from build123d import *

# Parameters (mm, degrees)
BOSS_EXTRUDE1_DEPTH = 2.5


with BuildPart() as part:
    # Sketch1 → Boss-Extrude1 (new, symmetric)
    with BuildSketch(Plane.XY):
        with BuildLine():
            Line((-25, 0), (-25, -40))
            Line((-25, -40), (25, -40))
            Line((25, -40), (25, 0))
            Line((25, 0), (18, 0))
            ThreePointArc((18, 0), (0, -18), (-18, 0))
            Line((-18, 0), (-25, 0))
        make_face()
    extrude(amount=BOSS_EXTRUDE1_DEPTH, both=True)


solid = part.part
Here's how the part is built. I have some questions about the finished solid (model axes, mm). Round coordinates to 2 decimals unless told otherwise and drop trailing zeros. Order: outer loops, then holes, each group sorted by start corner. A loop starts at its lowest first (then second) coordinate and runs counter-clockwise, first axis right, second up. Notation, with made-up numbers: (69, 19.25) -> (94, 19.25) arc R21 cw to (94, 28.25) -> close; hole circle Ø3 at (12, 46.5). An arc over 180 degrees is marked (long way). Return JSON: item names as keys, results as strings.
Q1. If we section it at B-B on z = -0.7: List the corners of the cut face in (x, y) for me, plus the area to 3 significant figures.
Filled sheet:
{"outline": "(-25, -40) -> (25, -40) -> (25, 0) -> (18, 0) arc R18 cw to (-18, 0) -> (-25, 0) -> close", "area": "1,490 mm^2"}
Q2. I need wall thicknesses on line 1 along X through (y, z) = (-8, 2); line 2 along X through (y, z) = (-15, 0.55); line 3 along Y through (x, z) = (-7.5, 0.8). Which ranges of each line are inside material? Lowest first, please. Write a range as from..to.
Filled sheet:
{"line 1": "x = -25..-16.12, 16.12..25", "line 2": "x = -25..-9.95, 9.95..25", "line 3": "y = -40..-16.36"}
Q3. If we section it at A-A on y = -13.5: List the corners of the cut face in (x, z) for me, plus the area to 3 significant figures.
Filled sheet:
{"outline": "(-25, -2.5) -> (-11.91, -2.5) -> (-11.91, 2.5) -> (-25, 2.5) -> close; (11.91, -2.5) -> (25, -2.5) -> (25, 2.5) -> (11.91, 2.5) -> close", "area": "131 mm^2"}
Q4. If we section it at D-D on y = -8.5: List the corners of the cut face in (x, z) for me.
Filled sheet:
{"outline": "(-25, -2.5) -> (-15.87, -2.5) -> (-15.87, 2.5) -> (-25, 2.5) -> close; (15.87, -2.5) -> (25, -2.5) -> (25, 2.5) -> (15.87, 2.5) -> close"}
Q5. If we section it at C-C on x = 0: List the corners of the cut face in (y, z) for me.
Filled sheet:
{"outline": "(-40, -2.5) -> (-18, -2.5) -> (-18, 2.5) -> (-40, 2.5) -> close"}
Q6. If we mould it in two halves opening along X, with no side actions, what happens to faces 1 (the cylindrical face through (0, -18, 0)), 2 (the flat face through (0, -24, -2.5)), 3 (the flat face through (-25, -20, 0))? For each: released by +X, released by -X, zero draft, split by the parting line, or undercut.
Filled sheet:
{"face 1": "undercut", "face 2": "zero draft", "face 3": "released by -X"}
